```python
from build123d import *

# Parameters (mm, degrees)
SKETCH1_W           = 190.5
SKETCH1_H           = 228.6
BOSS_EXTRUDE1_DEPTH = 6.35
CUT_EXTRUDE1_REACH  = 8.35


with BuildPart() as part:
    # Sketch1 → Boss-Extrude1 (new body)
    with BuildSketch(Plane(origin=(0, 0, 0), x_dir=(1, 0, 0), z_dir=(0, 1, 0))):
        Rectangle(SKETCH1_W, SKETCH1_H)
    extrude(amount=BOSS_EXTRUDE1_DEPTH)

    # Sketch2 → Cut-Extrude1 (cut, up to next)
    with BuildSketch(Plane(origin=(0, 6.35, 0), x_dir=(1, 0, 0), z_dir=(0, 1, 0)), mode=Mode.PRIVATE) as cut_extrude1_sk1:
        with BuildLine():
            Line((-7.112, 0), (-7.112, -38.1))
            ThreePointArc((-7.112, -38.1), (-9.906, -40.894), (-12.7, -38.1))
            Line((-12.7, -38.1), (-12.7, 0))
            ThreePointArc((-12.7, 0), (-9.906, 2.794), (-7.112, 0))
        make_face()
    cut_extrude1_tool1 = extrude(cut_extrude1_sk1.sketch, amount=-CUT_EXTRUDE1_REACH, mode=Mode.PRIVATE) & part.part
    add(cut_extrude1_tool1.solids().sort_by_distance((-9.906, 6.35, 19.05))[0], mode=Mode.SUBTRACT)
    # Sketch2 → Cut-Extrude1 (cut, up to next)
    with BuildSketch(Plane(origin=(0, 6.35, 0), x_dir=(1, 0, 0), z_dir=(0, 1, 0)), mode=Mode.PRIVATE) as cut_extrude1_sk2:
        with BuildLine():
            Line((13.208, 0), (13.208, -38.1))
            ThreePointArc((13.208, -38.1), (10.414, -40.894), (7.62, -38.1))
            Line((7.62, -38.1), (7.62, 0))
            ThreePointArc((7.62, 0), (10.414, 2.794), (13.208, 0))
        make_face()
    cut_extrude1_tool2 = extrude(cut_extrude1_sk2.sketch, amount=-CUT_EXTRUDE1_REACH, mode=Mode.PRIVATE) & part.part
    add(cut_extrude1_tool2.solids().sort_by_distance((10.414, 6.35, 19.05))[0], mode=Mode.SUBTRACT)


solid = part.part
```
Verification items for the finished model (mm, model axes). A direction names the side the tool comes from. Coordinates: 2 decimals unless noted, no trailing zeros. One line per question, with ' | ' between items. Start each with the question number.
1. Material ranges on line 1 along X through (y, z) = (5.75, 26.5), recorded low to high.
2. Access from +Z, -Z, +X, -X, +Y, -Y to the whole of each face (thin tool, end or side, straight path). Record for faces 4 (the flat face through (-1, 0, -2)), 5 (the flat face through (13.208, 3, 19)).
3. Draft check along X on faces 1 (the flat face through (95.25, 3, 2)), 2 (the cylindrical face through (10.475, 3.219, 40.893)), 3 (the flat face through (-1, 6.35, -2)). Enter one of: released by +X, released by -X, zero draft, split by the parting line, or undercut.
Computed values:
1) line 1: -95.25 to -12.7, -7.11 to 7.62, 13.21 to 95.25
2) face 4: +Z, -Z, +X, -X, -Y | face 5: +Y, -Y
3) face 1: released by +X | face 2: undercut | face 3: zero draft
